Can you work these out from the drawing? Everything is in mm from the part's minimum corner. Round coordinates to 2 decimals unless told otherwise and drop trailing zeros. Loops run counter-clockwise (first coordinate to the right, second up) from the corner with the lowest first, then second, coordinate; pieces in that order, holes last. Notation, with made-up numbers: (11, -21.5) -> (37, -21.5) arc R12 ccw to (37, -4.5) -> close; hole circle Ø1 at (83, -40). An arc over 180 degrees is marked (long way). One line per item, written item: value.
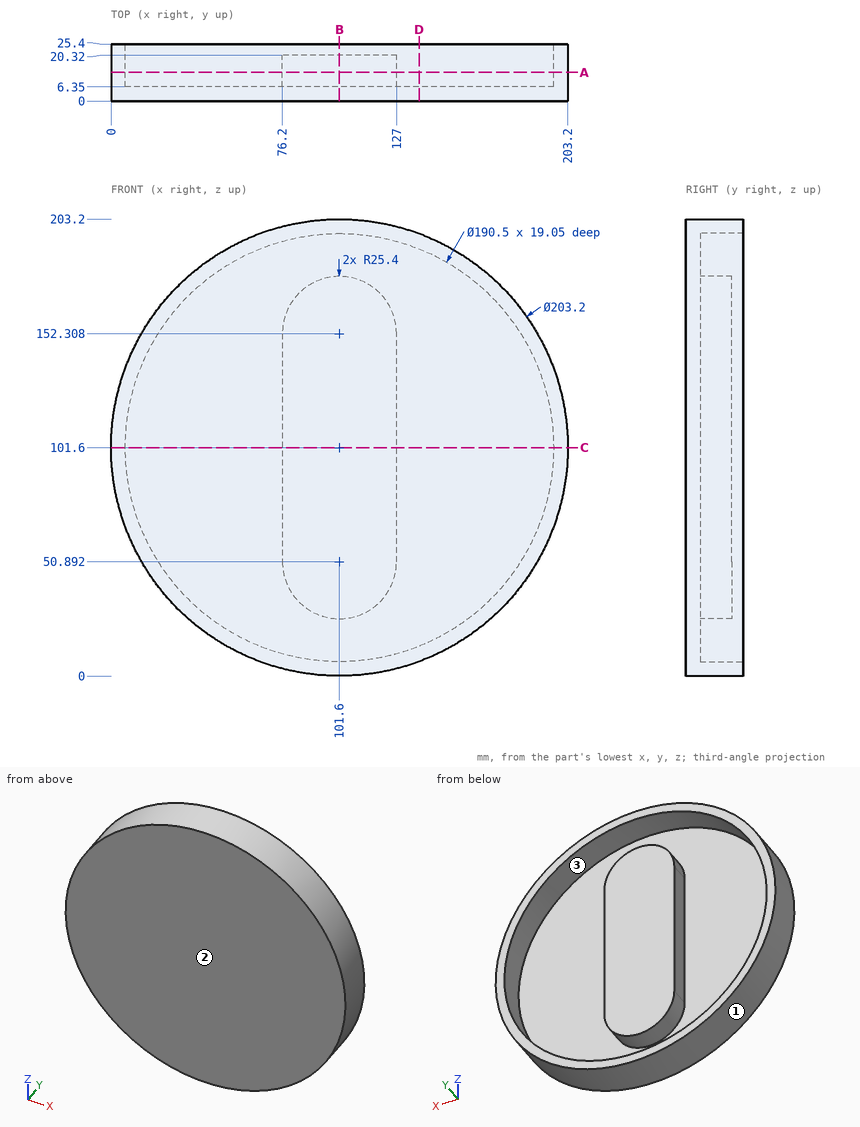
(1) Imagine slicing it at D-D on x = 137. Write out the boundary of the cut face in (y, z), then the cut area to 3 significant figures.
Results below:
outline: (0, 6.37) -> (25.4, 6.37) -> (25.4, 13.17) -> (6.35, 13.17) -> (6.35, 190.03) -> (25.4, 190.03) -> (25.4, 196.83) -> (0, 196.83) -> close
area: 1,470 mm²
(2) Imagine slicing it at A-A on y = 12.75. Write out the boundary of the cut face in (x, z).
Results below:
outline: circle Ø203.2 at (101.6, 101.6); (76.2, 50.89) arc R25.4 ccw to (127, 50.89) -> (127, 152.31) arc R25.4 ccw to (76.2, 152.31) -> close; hole circle Ø190.5 at (101.6, 101.6)
(3) We'd pull the mould along X, two halves only. Please class the marked faces 1, 2 and 3: +X half, -X half, draft (parallel to the pull), parting line (faces both ways), or undercut.
Results below:
face 1: parting line
face 2: draft
face 3: undercut
(4) Please list where these lines run through material, in increasing order: L1, parallel to X at y = 13.75, z = 101.6; L2, parallel to X at y = 8, z = 104.5; L3, parallel to Z at x = 114, y = 16.5.
Results below:
L1: x = 0 to 6.35, 76.2 to 127, 196.85 to 203.2
L2: x = 0.04 to 6.39, 76.2 to 127, 196.81 to 203.16
L3: z = 0.76 to 7.16, 28.72 to 174.48, 196.04 to 202.44
(5) Imagine slicing it at C-C on z = 101.6. Write out the boundary of the cut face in (x, y).
Results below:
outline: (0, 0) -> (203.2, 0) -> (203.2, 25.4) -> (196.85, 25.4) -> (196.85, 6.35) -> (127, 6.35) -> (127, 20.32) -> (76.2, 20.32) -> (76.2, 6.35) -> (6.35, 6.35) -> (6.35, 25.4) -> (0, 25.4) -> close
(6) Imagine slicing it at B-B on x = 101.6. Write out the boundary of the cut face in (y, z).
Results below:
outline: (0, 0) -> (25.4, 0) -> (25.4, 6.35) -> (6.35, 6.35) -> (6.35, 25.49) -> (20.32, 25.49) -> (20.32, 177.71) -> (6.35, 177.71) -> (6.35, 196.85) -> (25.4, 196.85) -> (25.4, 203.2) -> (0, 203.2) -> close
(7) For pin 1 Ø2 at (y, z) = (11, 85) entering from -X; pin 2 Ø12 at (x, y) = (21.5, 17) entering from +Z; pin 3 Ø3 at (x, z) = (31.5, 116) entering from +Y, each with a flat end and sliding along its axis, tell me the tip position at first contact or that it passes through.
Results below:
pin 1: stops at x = 1.2
pin 2: stops at z = 171.11
pin 3: stops at y = 6.35
